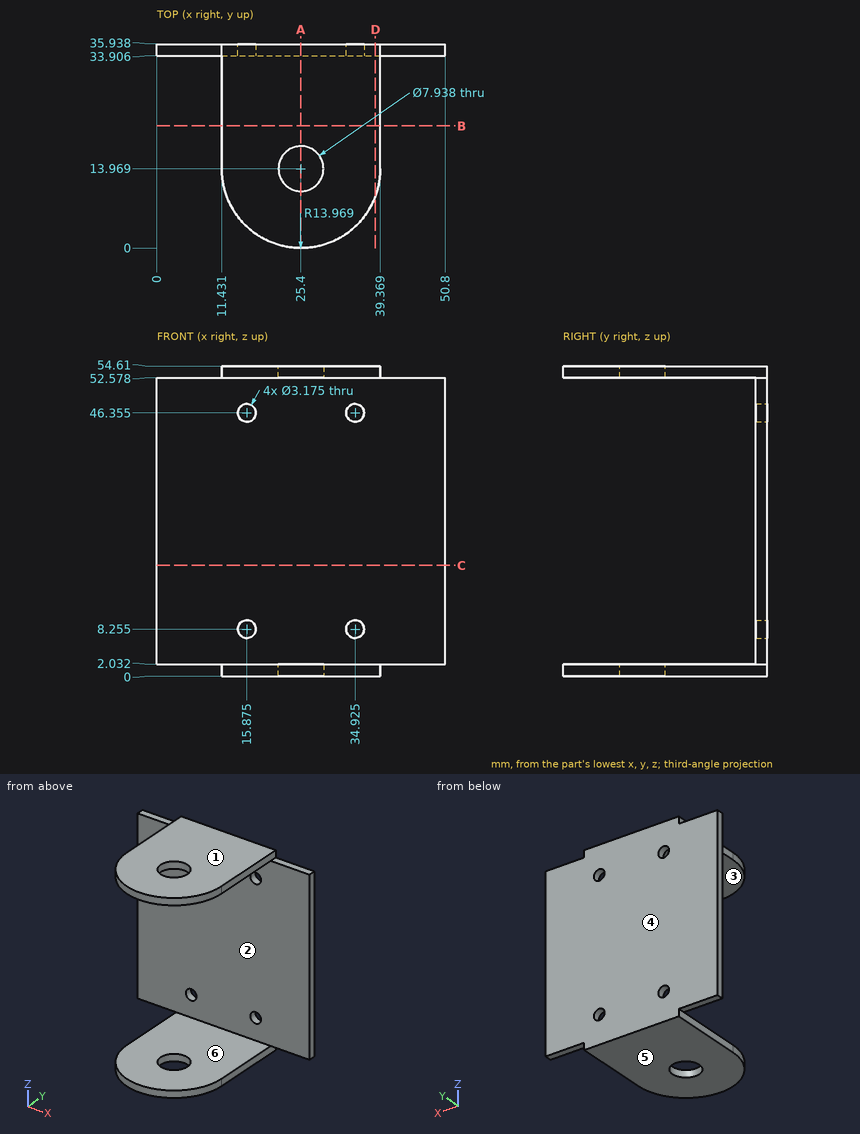
Geometry: see drawing. Coordinates: mm, zero at the bounding-box minimum. A direction names the side the tool comes from. Give positions to 0.01 mm unless a question says otherwise; leave off trailing zeros. Write each loop counter-clockwise with the first axis right and the second up, starting at its lowest first coordinate (ties: lowest second). Pieces come first, ordered by that corner, then holes. Notation, with made-up numbers: (47.5, -38) -> (106.5, -38) arc R20 cw to (106.5, -7) -> close; hole circle Ø1 at (-3.5, 67). An arc over 180 degrees is marked (long way). Use one line per item in the form item = value. Start each with the question number.
1) Section query B-B on y = 21.5. Return the cut outline in (x, z).
2) Set-up query: the marked faces 5 and 6. Return all of +Z, -Z, +X, -X, +Y, -Y with unobstructed straight access to the full face (end or side cutting, diameter ignored); none if empty.
3) Section query D-D on x = 38.5. Return the cut outline in (y, z) (1 decimal).
4) Section query C-C on z = 19.5. Return the cut outline in (x, y) (1 decimal).
5) Draft query along Z for the marked faces 1, 2, 3 and 4. Return one class per face: pulls with the +Z half, pulls with the -Z half, needs draft (parallel to the pull), parting line crosses it, or undercut.
6) Pin query (flat end, axial travel): pin 1 (1 mm diameter, centred on y = 20.5, z = 53.5, fed in from -X); pin 2 (0.6 mm diameter, centred on y = 20.5, z = 0.5, fed in from +X); pin 3 (1.9 mm diameter, centred on x = 15.875, z = 46.355, fed in from -Y) (3 decimals); pin 4 (0.6 mm diameter, centred on x = 45, y = 34.5, fed in from -Z). Return the tip coordinate at first contact, or that it passes through.
7) Section query A-A on x = 25.4. Return the cut outline in (y, z) (1 decimal).
8) Ray query, probe 1 along Y at (x, z) = (25.4, 53.4); probe 2 along Z at (x, y) = (16.5, 30); probe 3 along Y at (x, z) = (16, 44) (1 decimal). Return the intervals inside material, ascending. Write a range as from..to.
Outcome:
q1.outline = (11.43, 0) -> (39.37, 0) -> (39.37, 2.03) -> (11.43, 2.03) -> close; (11.43, 52.58) -> (39.37, 52.58) -> (39.37, 54.61) -> (11.43, 54.61) -> close
q2.face_5 = -Z, +X, -X, +Y, -Y
q2.face_6 = +X, -X, -Y
q3.outline = (9.1, 0) -> (35.9, 0) -> (35.9, 54.6) -> (9.1, 54.6) -> (9.1, 52.6) -> (33.9, 52.6) -> (33.9, 2) -> (9.1, 2) -> close
q4.outline = (0, 33.9) -> (50.8, 33.9) -> (50.8, 35.9) -> (0, 35.9) -> close
q5.face_1 = pulls with the +Z half
q5.face_2 = undercut
q5.face_3 = undercut
q5.face_4 = needs draft
q6.pin_1 = 11.43
q6.pin_2 = 39.37
q6.pin_3 = through
q6.pin_4 = 2.03
q7.outline = (0, 0) -> (10, 0) -> (10, 2) -> (0, 2) -> close; (0, 52.6) -> (10, 52.6) -> (10, 54.6) -> (0, 54.6) -> close; (17.9, 0) -> (35.9, 0) -> (35.9, 54.6) -> (17.9, 54.6) -> (17.9, 52.6) -> (33.9, 52.6) -> (33.9, 2) -> (17.9, 2) -> close
q8.probe_1 = 0..10, 17.94..35.94
q8.probe_2 = 0..2.03, 52.58..54.61
q8.probe_3 = 33.9..35.9
